Check sheet for the modelled part. Datum: model origin and axes. Units: mm. Give positions to 0.01 mm unless a question says otherwise; leave off trailing zeros. Write each loop counter-clockwise with the first axis right and the second up, starting at its lowest first coordinate (ties: lowest second). Pieces come first, ordered by that corner, then holes. Notation, with made-up numbers: M 27.5,66 L 42.5,66 A10 cw 42.5,72 Z; hole C -16.75,59 d7. An arc over 180 degrees is marked long. Use CSV: the item, a comma, the result in double quotes. Start each with the question number.
1. Cross-section at B-B, the plane x = -8.5. Enter the section's corners in (y, z).
2. Cross-section at A-A, the plane y = -158.5. Enter the section's corners in (x, z), and give its area (3 significant figures).
3. Scan lines: line 1 (Z direction, x = 10.5, y = 92.5); line 2 (Z direction, x = 10.5, y = -266); line 3 (X direction, y = 57.5, z = -12.5). Record each from-to range of solid material in increasing order.
4. Depth check by flat-ended pin: P1, Ø10, axis at x = 8, z = -13.5, coming from the +Y side; P2, Ø5, axis at y = -14, z = -45, coming from the +X side; P3, Ø1, axis at x = 8.5, z = -18, coming from the +Y side (3 decimals); P4, Ø3, axis at x = -9, y = 109, coming from the +Z side. Enter the tip coordinate at first touch or a pass-through.
5. Mould release check, pull along Z, two halves, no side actions. Record for faces 1 (the face through (7.313, 13.326, -15.331)), 2 (the face through (-12.7, 13, -1)), 3 (the face through (-3.13, 326.65, 2.47)): +Z half, -Z half, draft (parallel to the pull), parting line (faces both ways), or undercut.
from build123d import *

# Parameters (mm, degrees)
F0_W     = 25.4
F0_H     = 127
F1_DEPTH = 381
F2_SIZE  = 19.05
F4_DEPTH = 762.001
F6_DEPTH = 94.2936892712


with BuildPart() as f1:
    # F0 (on Front) → F1 (new body, symmetric)
    with BuildSketch(Plane.XZ):
        Rectangle(F0_W, F0_H)
    extrude(amount=F1_DEPTH, both=True)

    # F2
    f2_edges = [f1.edges().sort_by_distance(p)[0] for p in [
        (-12.7, 0, 63.5),
        (-12.7, 0, -63.5),
    ]]
    chamfer(f2_edges, length=F2_SIZE)

    # F3 (on face) → F4 (cut, through all)
    with BuildSketch(Plane.XZ.offset(381)):
        with BuildLine():
            ThreePointArc((11.0607444282, 37.7743444236), (12.2799882072, 35.3703719511), (12.7, 32.7078113162))
            Line((12.7, 32.7078113162), (12.7, 60.5742454254))
            ThreePointArc((12.7, 60.5742454254), (7.734521827, 49.4723711463), (11.0607444282, 37.7743444236))
        make_face()
        with BuildLine():
            ThreePointArc((12.7, 32.7078113162), (12.2050831664, 29.8239852054), (10.7769712009, 27.270185698))
            ThreePointArc((10.7769712009, 27.270185698), (6.7846666798, 15.7099875002), (11.1173224388, 4.2729961198))
            ThreePointArc((11.1173224388, 4.2729961198), (12.2916182124, 2.2783417271), (12.7, 0))
            Line((12.7, 0), (12.7, 32.7078113162))
        make_face()
        with BuildLine():
            Line((12.7, -31.8533331156), (12.7, 0))
            ThreePointArc((12.7, 0), (12.3437587955, -2.132292065), (11.3137291276, -4.0329803954))
            ThreePointArc((11.3137291276, -4.0329803954), (7.3105875393, -15.5042613468), (11.0984736295, -27.0484091373))
            ThreePointArc((11.0984736295, -27.0484091373), (12.2890761787, -29.3209339985), (12.7, -31.8533331156))
        make_face()
        with BuildLine():
            Line((12.7, -60.6248162719), (12.7, -31.8533331156))
            ThreePointArc((12.7, -31.8533331156), (11.8279315788, -35.4875740202), (9.4016464054, -38.3303456503))
            ThreePointArc((9.4016464054, -38.3303456503), (4.3012002964, -50.4761533584), (12.7, -60.6248162719))
        make_face()
    extrude(amount=-F4_DEPTH, mode=Mode.SUBTRACT)

    # F5 (on face) → F6 (cut, through all)
    with BuildSketch(Plane(origin=(-28.575, 0, 28.575), x_dir=(0, -1, 0), z_dir=(-0.7071067812, 0, 0.7071067812))):
        Polygon((381, 22.4506403027), (314.1107035763, 22.4506403027), (238.774623845, -52.8854394286), (381, -52.8854394286), align=None)
        Polygon((381, 49.3914086659), (341.0514719395, 49.3914086659), (314.1107035763, 22.4506403027), (381, 22.4506403027), align=None)
        Polygon((381, 53.8815367264), (345.5416, 53.8815367264), (341.0514719395, 49.3914086659), (381, 49.3914086659), align=None)
        Polygon((-349.5691035763, 22.4506403027), (-381, 22.4506403027), (-381, -78.4676751543), (-248.6507881192, -78.4676751543), align=None)
        Polygon((-376.5098719395, 49.3914086659), (-381, 49.3914086659), (-381, 22.4506403027), (-349.5691035763, 22.4506403027), align=None)
        Polygon((-376.5098719395, 49.3914086659), (-381, 53.8815367264), (-381, 49.3914086659), align=None)
    extrude(amount=-F6_DEPTH, mode=Mode.SUBTRACT)


solid = f1.part
Worked answers:
1,outline,"M -320.05,48.65 L -251.25,-48.65 L 286.71,-48.65 L 355.51,48.65 Z"
2,outline,"M -12.7,-44.45 L 6.35,-63.5 L 12.7,-63.5 L 12.7,-60.62 A12.72 cw 9.4,-38.33 A8.01 ccw 11.1,-27.05 A18.95 cw 11.31,-4.03 A6.56 ccw 11.12,4.27 A17.97 cw 10.78,27.27 A8.65 ccw 11.06,37.77 A17.79 cw 12.7,60.57 L 12.7,63.5 L 6.35,63.5 L -12.7,44.45 Z"
2,area,"2,410 mm^2"
3,line 1,"z = -63.5 to -59.61, -37.37 to -26.2, -5.16 to 5.03, 26.92 to 38.6, 57.8 to 63.5"
3,line 2,"z = -37.37 to -26.2, -5.16 to 5.03, 26.92 to 38.6, 57.8 to 63.5"
3,line 3,"x = -12.7 to 7.58"
4,P1,"stops at y = 327.23"
4,P2,"stops at x = 5.73"
4,P3,"passes through"
4,P4,"stops at z = 49.65"
5,face 1,"undercut"
5,face 2,"draft"
5,face 3,"-Z half"
